CAD build for the part. Positions are in the model's coordinates, mm. A direction names the side the tool comes from. Give positions to 0.01 mm unless a question says otherwise; leave off trailing zeros. Write each loop counter-clockwise with the first axis right and the second up, starting at its lowest first coordinate (ties: lowest second). Pieces come first, ordered by that corner, then holes. Notation, with made-up numbers: (79, -26) - (84, -26) arc R19 cw to (84, -6) - close; hole circle Ø10 at (24, 88.5). An arc over 180 degrees is marked (long way). Answer as a JSON object with one key per item and string values.
from build123d import *

# Parameters (mm, degrees)
F2_R    = 9.398
F4_R    = 7.62
F5_SIZE = 0.508


# Not quite as in the source:
# - a fillet or chamfer that OpenCascade refuses, or shapes differently, is made with other operations: its cross-section is extruded or revolved along the edge and cut away or added


with BuildPart() as f1:
    # F0 (on Front) → F1 (revolve)
    with BuildSketch(Plane.XZ):
        Polygon((0, 3.1496), (0, 0), (64.008, 0), (64.008, 9.4996), (8.001, 9.4996), (8.001, 3.1496), align=None)
    revolve(axis=Axis((-4.5283841901, 0, 0), (-1, 0, 0)))

    # F2
    f2_edges = [f1.edges().sort_by_distance(p)[0] for p in [
        (64.008, 0, -9.4996),
    ]]
    fillet(f2_edges, radius=F2_R)

    # F3: fillet of radius 7.62 on 1 edges, made by hand

    # F3_s1 → F3_t2 (revolve, cut)
    with BuildSketch(Plane.XZ):
        with BuildLine():
            ThreePointArc((15.5144213245, 9.4996), (10.5957324749, 7.6994711326), (8.001, 3.1496))
            Line((8.001, 3.1496), (8.001, 9.4996))
            Line((8.001, 9.4996), (15.5144213245, 9.4996))
        make_face()
    revolve(axis=Axis((8.001, 0, 0), (-1, 0, 0)), mode=Mode.SUBTRACT)

    # F4
    f4_edges = [f1.edges().sort_by_distance(p)[0] for p in [
        (8.001, 0, -3.1496),
    ]]
    fillet(f4_edges, radius=F4_R)

    # F5
    f5_edges = [f1.edges().sort_by_distance(p)[0] for p in [
        (0, 0, -3.1496),
    ]]
    chamfer(f5_edges, length=F5_SIZE)


solid = f1.part
(1) Saw through at A-A, the plane x = 24. Give the cut face in (y, z).
Answer key:
{"outline": "circle Ø19 at (0, 0)"}
(2) 3-axis set-ups, long thin cutter, end or side, ignore diameter. For faces 1 (the face through (1.8, -1.21, 2.91)), 2 (the face through (34.79, 6.42, -7)): which of +Z, -Z, +X, -X, +Y, -Y reach the whole face in a straight line?
Answer key:
{"face 1": "-X", "face 2": "+X, -X"}
(3) Flat gauge pins, fed straight in: P1, Ø2, axis at y = -2, z = -7.5, coming from the -X side; P2, Ø1.5, axis at x = 22, z = 5.5, coming from the +Y side; P3, Ø5, axis at x = 42.5, z = -5.5, coming from the -Y side. Where does each tip first touch, or does it go through?
Answer key:
{"P1": "stops at x = 9.66", "P2": "stops at y = 8.23", "P3": "stops at y = -9.01"}
(4) Probe L1, parallel to Y at x = 26, z = -0.25; L2, parallel to Z at x = 16.5, y = -1; L3, parallel to Y at x = 23.5, z = 5. List the from-to ranges inside material, lowest first. Write a range as [from, to].
Answer key:
{"L1": "y = [-9.5, 9.5]", "L2": "z = [-9.45, 9.45]", "L3": "y = [-8.08, 8.08]"}
